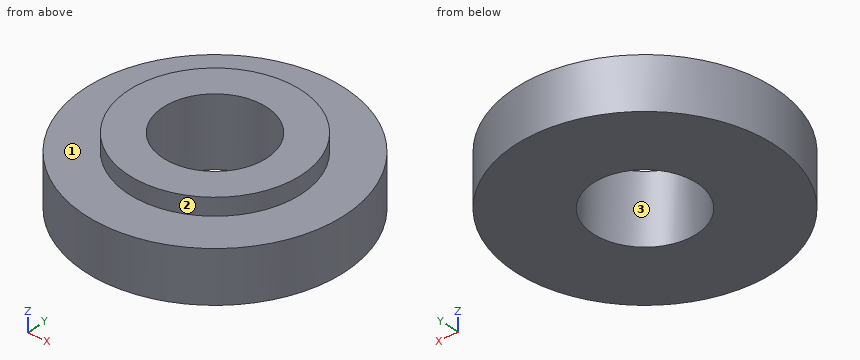
from build123d import *

# Parameters (mm, degrees)
SKETCH1_R           = 3.75
SKETCH1_R_2         = 1.5
BOSS_EXTRUDE1_DEPTH = 1.5
SKETCH2_R           = 2.5
SKETCH2_R_2         = 1.5
BOSS_EXTRUDE2_DEPTH = 0.5
SCALE1_SCALE        = 2


with BuildPart() as part:
    # Sketch1 → Boss-Extrude1 (new body)
    with BuildSketch(Plane.XY):
        Circle(SKETCH1_R)
        Circle(SKETCH1_R_2, mode=Mode.SUBTRACT)
    extrude(amount=BOSS_EXTRUDE1_DEPTH)

    # Sketch2 → Boss-Extrude2 (add)
    with BuildSketch(Plane.XY.offset(1.5)):
        Circle(SKETCH2_R)
        Circle(SKETCH2_R_2, mode=Mode.SUBTRACT)
    extrude(amount=BOSS_EXTRUDE2_DEPTH)


with BuildPart() as part_1:
    # Scale1: scaled about (0, 0, 0.851426307)
    add(part.part.scale(SCALE1_SCALE).moved(Location((0, 0, -0.851426307))))


solid = part_1.part
Read the model definition and answer for the solid it produces. Units are mm, in the model's axes. Face numbers are marked on the shaded views. Coordinates: 2 decimals unless noted, no trailing zeros. Order: outer loops, then holes, each group sorted by start corner. A loop starts at its lowest first (then second) coordinate and runs counter-clockwise, first axis right, second up. Notation, with made-up numbers: M -26,20 L 7,20 A26 ccw 7,36 Z; hole C 44,59.5 d10. An arc over 180 degrees is marked long. Put each result on its own line as item: value. Start each with the question number.
Item 1: Section D-D, the plane z = 0.5 is taken. Determine the outline of the cut face in (x, y), plus the area to 3 significant figures.
Item 2: Given pin 1 Ø3 at (x, y) = (5, -1.5) entering from +Z; pin 2 Ø5 at (x, y) = (0, 0) entering from -Z, each flat-ended and moving along its own axis, determine where each tip first touches the part or whether it passes through.
Item 3: Section A-A, the plane y = 0 is taken. Determine the outline of the cut face in (x, z), plus the area to 3 significant figures.
Item 4: Section C-C, the plane y = 3.75 is taken. Determine the outline of the cut face in (x, z).
Item 5: Consider probe 1 along Y at (x, z) = (0, 2.1); probe 2 along Y at (x, z) = (0, 2.2); probe 3 along Z at (x, y) = (6, 4.25). Determine where each line is inside the solid, lowest interval first. Write a range as [from, to].
Item 6: The mould has two halves that part along X. Classify the marked faces 1, 2 and 3: +X half, -X half, draft (parallel to the pull), parting line (faces both ways), or undercut.
Computed:
1. outline: C 0,0 d15; hole C 0,0 d6
1. area: 148 mm2
2. pin 1: stops at z = 3.15
2. pin 2: passes through
3. outline: M -7.5,-0.85 L -3,-0.85 L -3,3.15 L -5,3.15 L -5,2.15 L -7.5,2.15 Z; M 3,-0.85 L 7.5,-0.85 L 7.5,2.15 L 5,2.15 L 5,3.15 L 3,3.15 Z
3. area: 31.0 mm2
4. outline: M -6.5,-0.85 L 6.5,-0.85 L 6.5,2.15 L 3.31,2.15 L 3.31,3.15 L -3.31,3.15 L -3.31,2.15 L -6.5,2.15 Z
5. probe 1: y = [-7.5, -3], [3, 7.5]
5. probe 2: y = [-5, -3], [3, 5]
5. probe 3: z = [-0.85, 2.15]
6. face 1: draft
6. face 2: parting line
6. face 3: undercut
